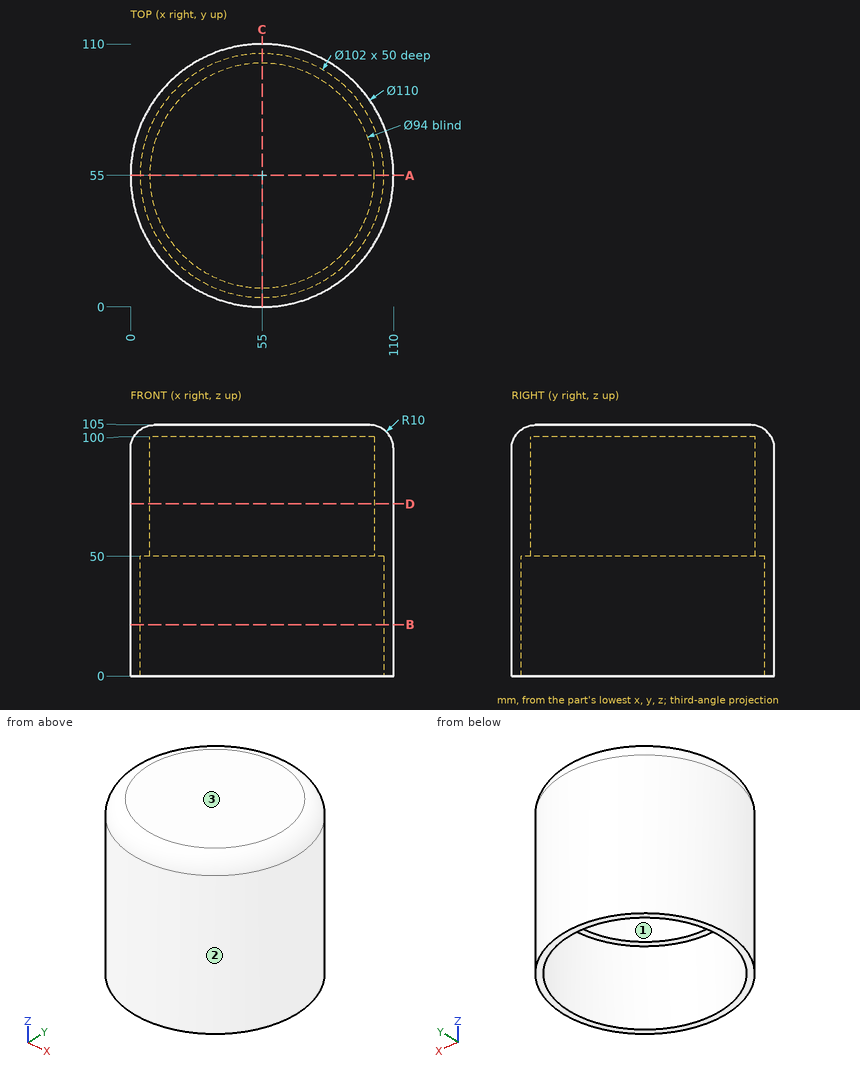
Design review of the part shown in the three views and the two pictorial views. Dimensions are in mm from the part's minimum x, y and z. Give positions to 0.01 mm unless a question says otherwise; leave off trailing zeros. Loops run counter-clockwise (first coordinate to the right, second up) from the corner with the lowest first, then second, coordinate; pieces in that order, holes last. Notation, with made-up numbers: (27, 24.25) - (70, 24.25) arc R24 cw to (70, 62.25) - close; hole circle Ø7 at (-1.75, -12.5). An arc over 180 degrees is marked (long way). Use CSV: the item, a comma, the result in double quotes. Start each with the question number.
1. Add section A-A (y = 55). State the section outline as (x, z) points.
2. Draft analysis for pull direction X (two halves, no side actions). For the marked faces 1, 2 and 3, state which applies: released by +X, released by -X, zero draft, split by the parting line, or undercut.
3. Add section B-B (z = 21.5). State the section outline as (x, y) points, plus the area to 3 significant figures.
4. Add section D-D (z = 72). State the section outline as (x, y) points.
5. Wall thickness on L1, parallel to Y at x = 55, z = 62; L2, parallel to Y at x = 55, z = 29; L3, parallel to Z at x = 44, y = 81: over which ranges is each line inside the solid? List them lowest first.
6. Insertion check: P1, Ø10, axis at x = 25, z = 51, coming from the +Y side; P2, Ø2, axis at y = 31.5, z = 67, coming from the +X side; P3, Ø10, axis at x = 52, y = 52.5, coming from the -Z side. Each pin has a flat end and moves straight along its axis. Give the tip position at first contact, or say it passes through.
Results found:
1,outline,"(0, 0) - (4, 0) - (4, 50) - (8, 50) - (8, 100) - (102, 100) - (102, 50) - (106, 50) - (106, 0) - (110, 0) - (110, 95) arc R10 ccw to (100, 105) - (10, 105) arc R10 ccw to (0, 95) - close"
2,face 1,"undercut"
2,face 2,"split by the parting line"
2,face 3,"zero draft"
3,outline,"circle Ø110 at (55, 55); hole circle Ø102 at (55, 55)"
3,area,"1,330 mm²"
4,outline,"circle Ø110 at (55, 55); hole circle Ø94 at (55, 55)"
5,L1,"y = 0 to 8, 102 to 110"
5,L2,"y = 0 to 4, 106 to 110"
5,L3,"z = 100 to 105"
6,P1,"stops at y = 103.99"
6,P2,"stops at x = 105.19"
6,P3,"stops at z = 100"
